The model under review builds one solid part; all positions refer to its coordinate system, in mm. Round coordinates to 2 decimals unless told otherwise and drop trailing zeros. Order: outer loops, then holes, each group sorted by start corner. A loop starts at its lowest first (then second) coordinate and runs counter-clockwise, first axis right, second up. Notation, with made-up numbers: M -20.75,-14.75 L 24.25,-14.75 A27 ccw 24.25,19.25 Z; hole C -36.5,74 d8. An arc over 180 degrees is marked long. One line per item, written item: value. Start each with the question number.
from build123d import *

# Parameters (mm, degrees)
F0_W     = 130.198062
F0_H     = 64.74135
F1_DEPTH = 25.4
F3_R     = 17.084004
F4_DEPTH = 25.4
F6_DEPTH = 56.896


with BuildPart() as f1:
    # F0 (on Top) → F1 (new body)
    with BuildSketch(Plane.XY):
        Rectangle(F0_W, F0_H)
    extrude(amount=F1_DEPTH)

    # F3 (on face) → F4 (join)
    with BuildSketch(Plane.XY.offset(25.4)):
        Circle(F3_R)
    extrude(amount=F4_DEPTH)

    # F5 (on Front) → F6 (cut, symmetric)
    with BuildSketch(Plane.XZ):
        Polygon((17.084004, 50.8), (-17.084004, 50.8), (17.084004, 25.4), align=None)
    extrude(amount=F6_DEPTH, both=True, mode=Mode.SUBTRACT)


solid = f1.part
Item 1: Consider section A-A, the plane x = 0. Give the boundary of the cut face in (y, z), then the cut area to 3 significant figures.
Item 2: Consider section C-C, the plane z = 39.5. Give the boundary of the cut face in (x, y), then the cut area to 3 significant figures.
Item 3: Consider section B-B, the plane y = 10.5. Give the boundary of the cut face in (x, z), then the cut area to 3 significant figures.
Item 4: Clearance check with flat-ended pins moving along their axes: P1, Ø19.5, axis at x = -16, y = -14.5, coming from the +Z side; P2, Ø4, axis at x = -11.5, z = 41, coming from the -Y side; P3, Ø3, axis at x = -10, z = 34, coming from the +Y side. State where each tip first meets the part, or that it passes through.
Item 5: Wall thickness on L1, parallel to Z at x = -30.5, y = -6.5; L2, parallel to X at y = 5, z = 42.5; L3, parallel to X at y = 12.5, z = 26: over which ranges is each line inside the solid? List them lowest first.
Item 6: Consider section D-D, the plane x = -23. Give the boundary of the cut face in (y, z).
Computed:
1. outline: M -32.37,0 L 32.37,0 L 32.37,25.4 L 17.08,25.4 L 17.08,38.1 L -17.08,38.1 L -17.08,25.4 L -32.37,25.4 Z
1. area: 2,080 mm^2
2. outline: M -1.88,-16.98 L -1.88,16.98 A17.08 ccw Z
2. area: 394 mm^2
3. outline: M -65.1,0 L 65.1,0 L 65.1,25.4 L 13.48,25.4 L 13.48,28.08 L -13.48,48.12 L -13.48,25.4 L -65.1,25.4 Z
3. area: 3,650 mm^2
4. P1: stops at z = 50.3
4. P2: stops at y = -14.2
4. P3: stops at y = 14.82
5. L1: z = 0 to 25.4
5. L2: x = -16.34 to -5.92
5. L3: x = -11.65 to 11.65
6. outline: M -32.37,0 L 32.37,0 L 32.37,25.4 L -32.37,25.4 Z
